from build123d import *

# Parameters (mm, degrees)
SKETCH1_W           = 107
SKETCH1_H           = 4
BOSS_EXTRUDE1_DEPTH = 55
SKETCH2_W           = 15
SKETCH2_H           = 4
BOSS_EXTRUDE2_DEPTH = 4


with BuildPart() as part:
    # Sketch1 → Boss-Extrude1 (new body)
    with BuildSketch(Plane(origin=(0, 0, 0), x_dir=(1, 0, 0), z_dir=(0, 1, 0))):
        Rectangle(SKETCH1_W, SKETCH1_H)
    extrude(amount=BOSS_EXTRUDE1_DEPTH)

    # Sketch2 → Boss-Extrude2 (add)
    with BuildSketch(Plane.XZ):
        with Locations((-30, 0)):
            Rectangle(SKETCH2_W, SKETCH2_H)
        Rectangle(SKETCH2_W, SKETCH2_H)
        with Locations((30, 0)):
            Rectangle(SKETCH2_W, SKETCH2_H)
    extrude(amount=BOSS_EXTRUDE2_DEPTH)


solid = part.part
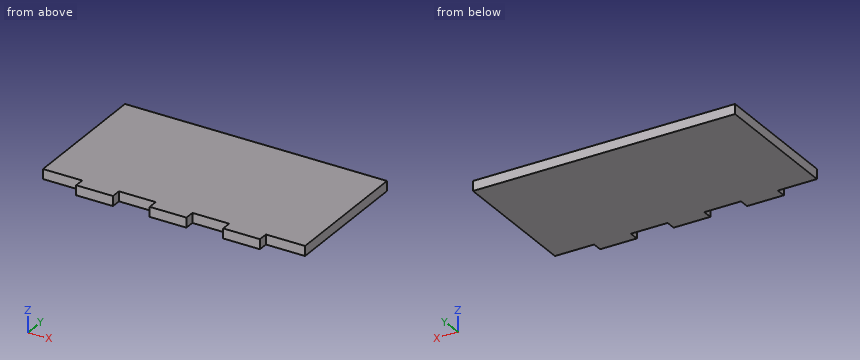
Geometry check sheet. Reference: the model listing, model coordinates, mm. Round coordinates to 2 decimals unless told otherwise and drop trailing zeros. Write each loop counter-clockwise with the first axis right and the second up, starting at its lowest first coordinate (ties: lowest second). Pieces come first, ordered by that corner, then holes. Notation, with made-up numbers: (-29, 32.5) -> (-22, 32.5) arc R12 ccw to (-22, 46.5) -> close; hole circle Ø7 at (-25.5, 77). An arc over 180 degrees is marked (long way). One line per item, written item: value. Start each with the question number.
(1) Scan line: line 1 (Y direction, x = 18.5, z = -1.5). Record every from-to range of solid material in increasing order. Write a range as [from, to].
(2) Cross-section at B-B, the plane x = -11. Record the cut outline in (y, z).
(3) Go/stop test with flat-tipped pins: pin 1 Ø2 at (x, z) = (-16, 0) entering from -Y; pin 2 Ø2 at (y, z) = (-2, 0) entering from +X; pin 3 Ø1.2 at (y, z) = (-1.5, -1) entering from -X. Record where each tip stops, or that it passes through.
(4) Cross-section at A-A, the plane z = 1. Record the cut outline in (x, y).
Answer:
1. line 1: [0, 55]
2. outline: (0, -2) -> (55, -2) -> (55, 2) -> (0, 2) -> close
3. pin 1: y = 0
3. pin 2: x = 37.5
3. pin 3: x = -37.5
4. outline: (-53.5, 0) -> (-37.5, 0) -> (-37.5, -4) -> (-22.5, -4) -> (-22.5, 0) -> (-7.5, 0) -> (-7.5, -4) -> (7.5, -4) -> (7.5, 0) -> (22.5, 0) -> (22.5, -4) -> (37.5, -4) -> (37.5, 0) -> (53.5, 0) -> (53.5, 55) -> (-53.5, 55) -> close
